Design review of the part built by this model. Coordinates are the model's own, in mm. Face numbers are marked on the shaded views. A direction names the side the tool comes from. Coordinates: 2 decimals unless noted, no trailing zeros. Order: outer loops, then holes, each group sorted by start corner. A loop starts at its lowest first (then second) coordinate and runs counter-clockwise, first axis right, second up. Notation, with made-up numbers: M 34,-4 L 73,-4 A25 ccw 73,19 Z; hole C -37,15.5 d9. An arc over 180 degrees is marked long. Answer in a Markdown table with one row per item.
from build123d import *

# Parameters (mm, degrees)
F0_W            = 150
F0_H            = 55
F0_W_2          = 144
F0_H_2          = 49
F1_DEPTH        = 20
F3_R            = 4.75
F4_DEPTH        = 25
F5_W            = 8
F5_H            = 19.383624
F6_DEPTH        = 20
F8_DEPTH        = 25
F2_R            = 4.75
F9_DEPTH        = 3
F10_R           = 2
F12_DEPTH       = 56
F13_W           = 30
F13_H           = 56
F14_DEPTH       = 25
F16_DEPTH       = 3
F17_R           = 6
F17_R_2         = 4.92693
F18_DEPTH       = 25
F19_R           = 1.25
F20_DEPTH       = 10
F21_R           = 1.75
F22_DEPTH       = 10
F24_D           = 3
F24_CSINK_D     = 8
F24_CSINK_ANGLE = 90
F26_DEPTH       = 45.981508
F28_DEPTH       = 82.704807
F30_DEPTH       = 3.001
F32_DEPTH       = 3


with BuildPart() as f1:
    # F0 (on Top) → F1 (new body)
    with BuildSketch(Plane.XY):
        with Locations((75, 0)):
            Rectangle(F0_W, F0_H)
        with Locations((75, 0)):
            Rectangle(F0_W_2, F0_H_2, mode=Mode.SUBTRACT)
    extrude(amount=F1_DEPTH)

    # F3 (on Top) → F4 (cut)
    with BuildSketch(Plane.XY):
        with Locations((55.75, 30)):
            Circle(F3_R)
        with Locations((55.75, -30)):
            Circle(F3_R)
    extrude(amount=F4_DEPTH, mode=Mode.SUBTRACT)

    # F5 (on Top) → F6 (join)
    with BuildSketch(Plane.XY):
        with Locations((136, 35.308188)):
            Rectangle(F5_W, F5_H)
        with Locations((136, -35.308188)):
            Rectangle(F5_W, F5_H)
    extrude(amount=F6_DEPTH)

    # F7 (on face) → F8 (cut)
    with BuildSketch(Plane.YZ.offset(140)):
        with BuildLine():
            Line((45, 20), (27.5, 20))
            ThreePointArc((27.5, 20), (34.452449, 10.753061), (45, 6))
            Line((45, 6), (45, 20))
        make_face()
        with BuildLine():
            Line((-27.5, 20), (-45, 20))
            Line((-45, 20), (-45, 6))
            ThreePointArc((-45, 6), (-34.452449, 10.753061), (-27.5, 20))
        make_face()
    extrude(amount=-F8_DEPTH, mode=Mode.SUBTRACT)

    # F2 (on Top) → F9 (join)
    with BuildSketch(Plane.XY):
        with BuildLine():
            Line((45.902228, 27.5), (0, 27.5))
            Line((0, 27.5), (0, -27.5))
            Line((0, -27.5), (45.902228, -27.5))
            ThreePointArc((45.902228, -27.5), (55.75, -40.160149), (65.597772, -27.5))
            Line((65.597772, -27.5), (150, -27.5))
            Line((150, -27.5), (150, 27.5))
            Line((150, 27.5), (65.597772, 27.5))
            ThreePointArc((65.597772, 27.5), (55.75, 40.160149), (45.902228, 27.5))
        make_face()
        with Locations((55.75, -30)):
            Circle(F2_R, mode=Mode.SUBTRACT)
        with Locations((55.75, 30)):
            Circle(F2_R, mode=Mode.SUBTRACT)
    extrude(amount=F9_DEPTH)

    # F10
    f10_edges = [f1.edges().sort_by_distance(p)[0] for p in [
        (51, 30, 0),
        (51, -30, 0),
    ]]
    fillet(f10_edges, radius=F10_R)

    # F11 (on face) → F12 (join)
    with BuildSketch(Plane.XY.offset(3)):
        Polygon((45.981508, 27.601903), (0, 27.601903), (0, 0), (0, -27.601903), (45.981508, -27.601903), (45.981508, -24.5), (3, -24.5), (3, 0), (3, 24.5), (45.981508, 24.5), align=None)
    extrude(amount=F12_DEPTH)

    # F13 (on face) → F14 (cut)
    with BuildSketch(Plane(origin=(0, 0, 0), x_dir=(0, -1, 0), z_dir=(-1, 0, 0))):
        with Locations((0, 31)):
            Rectangle(F13_W, F13_H)
    extrude(amount=-F14_DEPTH, mode=Mode.SUBTRACT)

    # F15 (on face) → F16 (join)
    with BuildSketch(Plane.XY.offset(59)):
        Polygon((0, 15), (3, 15), (14.855375, 24.5), (14.855375, 27.601903), (0, 27.601903), align=None)
        Polygon((3, -15), (0, -15), (0, -27.601903), (14.855375, -27.601903), (14.855375, -24.5), align=None)
    extrude(amount=F16_DEPTH)

    # F17 (on face) → F18 (cut)
    with BuildSketch(Plane.XY.offset(3)):
        with Locations((15.74922, 0)):
            Circle(F17_R)
        with Locations((40.74922, 0)):
            Circle(F17_R)
        with Locations((65.74922, 0)):
            Circle(F17_R)
        with Locations((90.74922, 0)):
            Circle(F17_R)
        with Locations((115.74922, 0)):
            Circle(F17_R)
        with Locations((28.24922, 14)):
            Circle(F17_R_2)
        with Locations((53.24922, 14)):
            Circle(F17_R_2)
        with Locations((78.24922, 14)):
            Circle(F17_R_2)
        with Locations((103.24922, 14)):
            Circle(F17_R_2)
        with Locations((128.24922, 14)):
            Circle(F17_R_2)
        with Locations((28.24922, -14)):
            Circle(F17_R_2)
        with Locations((53.24922, -14)):
            Circle(F17_R_2)
        with Locations((78.24922, -14)):
            Circle(F17_R_2)
        with Locations((103.24922, -14)):
            Circle(F17_R_2)
        with Locations((128.24922, -14)):
            Circle(F17_R_2)
    extrude(amount=-F18_DEPTH, mode=Mode.SUBTRACT)

    # F19 (on face) → F20 (cut)
    with BuildSketch(Plane.XZ.offset(45)):
        with Locations((136, 3)):
            Circle(F19_R)
    extrude(amount=-F20_DEPTH, mode=Mode.SUBTRACT)

    # F21 (on face) → F22 (cut)
    with BuildSketch(Plane(origin=(0, 45, 0), x_dir=(-1, 0, 0), z_dir=(0, 1, 0))):
        with Locations((-136, 3)):
            Circle(F21_R)
    extrude(amount=-F22_DEPTH, mode=Mode.SUBTRACT)

    # F24 (through all)
    with Locations(Plane.XY.offset(3)):
        with Locations((12.257308, 14.712964), (12.257308, -14.712964)):
            CounterSinkHole(F24_D / 2, F24_CSINK_D / 2, counter_sink_angle=F24_CSINK_ANGLE)

    # F25 (on face) → F26 (join, through all)
    with BuildSketch(Plane(origin=(0, 0, 0), x_dir=(0, -1, 0), z_dir=(-1, 0, 0))):
        Polygon((-55.101903, 44), (-55.101903, 38), (-41.280588, 38), (-27.601903, 36.453437), (-27.601903, 40), (-53.101903, 40), (-53.101903, 44), align=None)
        Polygon((-55.101903, 24), (-55.101903, 18), (-34.022562, 18), (-27.601903, 14.44634), (-27.601903, 20), (-53.101903, 20), (-53.101903, 24), align=None)
        Polygon((55.101903, 24), (53.101903, 24), (53.101903, 20), (27.601903, 20), (27.601903, 14.44634), (34.022562, 18), (55.101903, 18), align=None)
        Polygon((41.280588, 38), (55.101903, 38), (55.101903, 44), (53.101903, 44), (53.101903, 40), (27.601903, 40), (27.601903, 36.453437), align=None)
    extrude(amount=-F26_DEPTH)

    # F27 (on face) → F28 (cut, through all)
    with BuildSketch(Plane.XZ.offset(27.601903)):
        with BuildLine():
            Line((45.981508, 59), (14.855375, 59))
            ThreePointArc((14.855375, 59), (29.645011, 50.637717), (45.981508, 45.970812))
            Line((45.981508, 45.970812), (45.981508, 59))
        make_face()
    extrude(amount=-F28_DEPTH, mode=Mode.SUBTRACT)

    # F29 (on face) → F30 (cut, through all)
    with BuildSketch(Plane.XY.offset(3)):
        with BuildLine():
            Line((15.681136, 6.499643), (15.817265, 6.499644))
            ThreePointArc((15.817265, 6.499644), (15.7492, 6.5), (15.681136, 6.499643))
        make_face()
        with BuildLine():
            Line((134.703036, 6.5), (15.817265, 6.499644))
            Line((15.817265, 6.499644), (15.681136, 6.499643))
            ThreePointArc((15.681136, 6.499643), (9.249862, -0.091384), (15.863902, -6.498988))
            Line((15.863902, -6.498988), (134.703, -6.5))
            ThreePointArc((134.703, -6.5), (141.203055, -1.8e-05), (134.703036, 6.5))
        make_face()
    extrude(amount=-F30_DEPTH, mode=Mode.SUBTRACT)

    # F31 (on face) → F32 (join)
    with BuildSketch(Plane.XY):
        Polygon((139.584467, -37.202392), (149.647281, -27.13958), (123.585731, -27.196111), (132.348284, -37.202392), align=None)
        Polygon((149.647281, 27.13958), (139.584467, 37.202392), (132.348284, 37.202392), (123.585731, 27.196111), align=None)
    extrude(amount=F32_DEPTH)


solid = f1.part
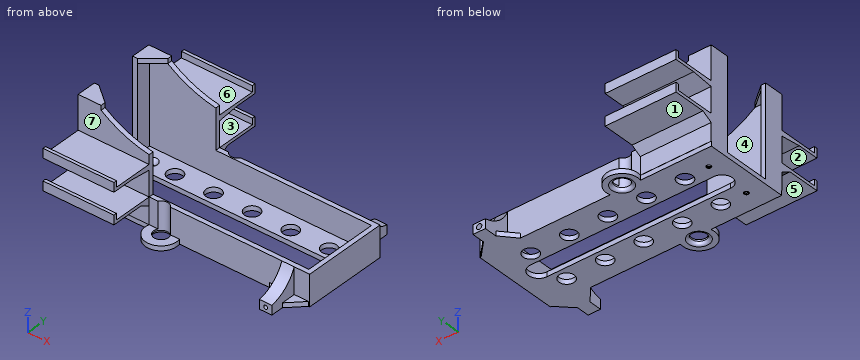
(1) For line 1 along Y through (x, z) = (37, 21); line 2 along Z through (x, y) = (30.5, -45); line 3 along X through (y, z) = (-23.5, 12), list the stretches that pass through material, from the lowest coordinate up. Write a range as from..to.
Return value:
| item | result |
|---|---|
| line 1 | y = -55.1..-53.1, -27.6..-24.5, 24.5..27.6, 53.1..55.1 |
| line 2 | z = 18..20, 38..40 |
| line 3 | x = 0..3, 147..150 |
(2) For the marked faces 1, 2 and 3, list the 3-axis set-ups (+Z, -Z, +X, -X, +Y, -Y) from which the entire face can be reached by the end or side of a thin tool; tool diameter is ignored.
Return value:
| item | result |
|---|---|
| face 1 | -Z, +X, -X, +Y |
| face 2 | +X, -X, -Y |
| face 3 | +X, -X |
(3) Draft analysis for pull direction Z (two halves, no side actions). For the marked faces 4, 5, 6 and 7, state which applies: pulls with the +Z half, pulls with the -Z half, needs draft (parallel to the pull), parting line crosses it, or undercut.
Return value:
| item | result |
|---|---|
| face 4 | undercut |
| face 5 | pulls with the -Z half |
| face 6 | pulls with the +Z half |
| face 7 | needs draft |
(4) Insertion check: pin 1 Ø3 at (x, z) = (18.5, 51) entering from -Y; pin 2 Ø6.5 at (x, y) = (32, 49) entering from -Z; pin 3 Ø12 at (x, y) = (18.5, -7.5) entering from +Z. Each pin has a flat end and moves straight along its axis. Give the tip position at first contact, or say it passes through.
Return value:
| item | result |
|---|---|
| pin 1 | stops at y = -27.6 |
| pin 2 | stops at z = 18 |
| pin 3 | stops at z = 3 |
(5) Add section B-B, the plane z = 33.5. Give the boundary of the cut face in (x, y), and give its area (3 significant figures).
Return value:
| item | result |
|---|---|
| outline | M 0,-27.6 L 45.98,-27.6 L 45.98,-24.5 L 3,-24.5 L 3,-15 L 0,-15 Z; M 0,15 L 3,15 L 3,24.5 L 45.98,24.5 L 45.98,27.6 L 0,27.6 Z |
| area | 342 mm2 |
(6) Add section A-A, the plane y = 0. Give the boundary of the cut face in (x, z), and give its area (3 significant figures).
Return value:
| item | result |
|---|---|
| outline | M 0,0 L 9.25,0 L 9.25,3 L 0,3 Z; M 141.2,0 L 150,0 L 150,20 L 147,20 L 147,3 L 141.2,3 Z |
| area | 105 mm2 |
(7) Add section C-C, the plane x = 69. Give the boundary of the cut face in (y, z).
Return value:
| item | result |
|---|---|
| outline | M -27.5,0 L -6.5,0 L -6.5,3 L -24.5,3 L -24.5,20 L -27.5,20 Z; M 6.5,0 L 27.5,0 L 27.5,20 L 24.5,20 L 24.5,3 L 6.5,3 Z |
(8) Add section D-D, the plane y = -30. Give the boundary of the cut face in (x, z), and give its area (3 significant figures).
Return value:
| item | result |
|---|---|
| outline | M 0,15.77 L 45.98,15.77 L 45.98,20 L 0,20 Z; M 0,36.72 L 45.98,36.72 L 45.98,40 L 0,40 Z; M 45.59,0 L 49,0 A2 ccw 51,2 L 51,3 L 45.59,3 Z; M 60.5,2 A2 ccw 62.5,0 L 65.91,0 L 65.91,3 L 60.5,3 Z; M 126.04,0 L 146.79,0 L 146.79,3 L 140,3 L 140,15.47 L 132,15.47 L 132,3 L 126.04,3 Z |
| area | 538 mm2 |
